For this review, use the dimensioned drawing (mm, ordinates from the lowest corner) and the shaded views. Round coordinates to 2 decimals unless told otherwise and drop trailing zeros. Order: outer loops, then holes, each group sorted by start corner. A loop starts at its lowest first (then second) coordinate and runs counter-clockwise, first axis right, second up. Notation, with made-up numbers: (58, -3) - (99, -3) arc R15 ccw to (99, 6) - close; hole circle Ø6 at (44, -25). An arc over 180 degrees is marked (long way). Write each question's results on one line, items separated by ' | '. Start each with the question number.
(1) Take a section at C-C, the plane z = 1.85. Give the boundary of the cut face in (x, y), plus the area to 3 significant figures.
(2) Take a section at A-A, the plane y = 18. Give the boundary of the cut face in (x, z).
(3) For L1, parallel to Y at x = 228.5, z = 1.6; L2, parallel to X at y = 17, z = 1.9; L3, parallel to Y at x = 248, z = 2.8, list the stretches that pass through material, from the lowest coordinate up. Write a range as from..to.
(4) Insertion check: pin 1 Ø1 at (x, z) = (176, 2) entering from -Y; pin 2 Ø3.5 at (x, y) = (58.5, 18) entering from -Z; pin 3 Ø0.9 at (y, z) = (2, 1.5) entering from -X; pin 4 Ø1.5 at (y, z) = (1, 1.5) entering from +X. Each pin has a flat end and moves straight along its axis. Give the tip position at first contact, or say it passes through.
(5) Take a section at B-B, the plane x = 58.5. Give the boundary of the cut face in (y, z), plus the area to 3 significant figures.
(6) Take a section at D-D, the plane x = 93. Give the boundary of the cut face in (y, z).
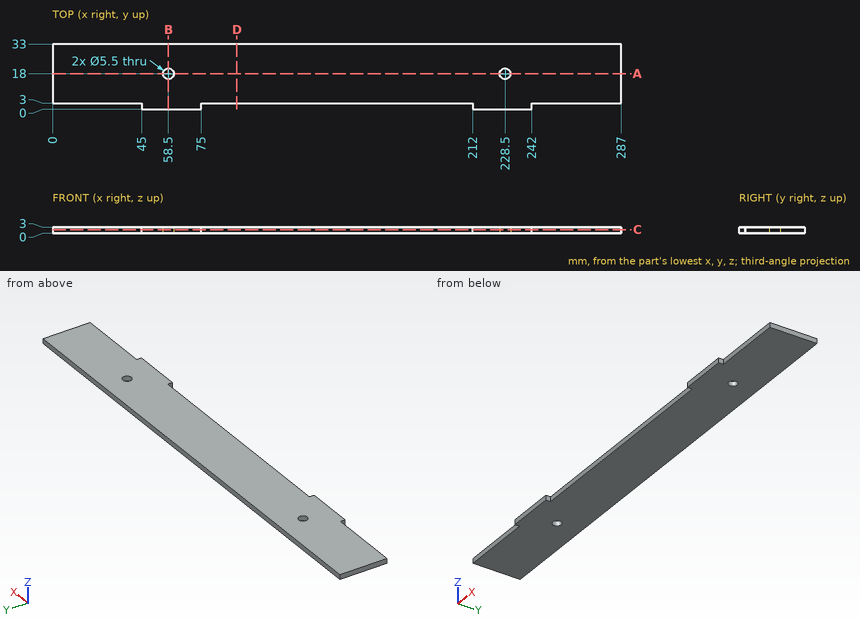
Results below:
1) outline: (0, 3) - (45, 3) - (45, 0) - (75, 0) - (75, 3) - (212, 3) - (212, 0) - (242, 0) - (242, 3) - (287, 3) - (287, 33) - (0, 33) - close; hole circle Ø5.5 at (58.5, 18); hole circle Ø5.5 at (228.5, 18) | area: 8,740 mm^2
2) outline: (0, 0) - (55.75, 0) - (55.75, 3) - (0, 3) - close; (61.25, 0) - (225.75, 0) - (225.75, 3) - (61.25, 3) - close; (231.25, 0) - (287, 0) - (287, 3) - (231.25, 3) - close
3) L1: y = 0..15.25, 20.75..33 | L2: x = 0..55.94, 61.06..225.94, 231.06..287 | L3: y = 3..33
4) pin 1: stops at y = 3 | pin 2: passes through | pin 3: stops at x = 45 | pin 4: stops at x = 242
5) outline: (0, 0) - (15.25, 0) - (15.25, 3) - (0, 3) - close; (20.75, 0) - (33, 0) - (33, 3) - (20.75, 3) - close | area: 82.5 mm^2
6) outline: (3, 0) - (33, 0) - (33, 3) - (3, 3) - close
